from build123d import *

# Parameters (mm, degrees)
SKETCH_R     = 8.5
PAD_DEPTH    = 38
SKETCH001_R  = 4.6
PAD001_DEPTH = 10
FILLET_R     = 1


with BuildPart() as part:
    # Sketch → Pad (new body)
    with BuildSketch(Plane.XY):
        Circle(SKETCH_R)
    extrude(amount=PAD_DEPTH)

    # Sketch001 (on Face2 of Pad) → Pad001 (join)
    with BuildSketch(Plane(origin=(0, 0, 0), x_dir=(1, 0, 0), z_dir=(0, 0, -1))):
        Circle(SKETCH001_R)
    extrude(amount=PAD001_DEPTH)

    # Fillet
    fillet_edges = [part.edges().sort_by_distance(p)[0] for p in [
        (-4.6, 0, -10),
        (-8.5, 0, 0),
    ]]
    fillet(fillet_edges, radius=FILLET_R)


solid = part.part
Build history of the part. All positions in model axes, mm. A direction names the side the tool comes from. Round coordinates to 2 decimals unless told otherwise and drop trailing zeros. Write each loop counter-clockwise with the first axis right and the second up, starting at its lowest first coordinate (ties: lowest second). Pieces come first, ordered by that corner, then holes. Notation, with made-up numbers: M 28.5,79.5 L 66.5,79.5 A26 ccw 66.5,115.5 Z; hole C -36,50 d5. An arc over 180 degrees is marked long. Answer as a JSON object with one key per item and string values. Group by question number.
(1) Cut at C-C (z = 10). Give the cut face in (x, y), and give its area (3 significant figures).
(2) Which spindle directions (+Z, -Z, +X, -X, +Y, -Y) get a long thin tool onto all of the face, cutting with end or side? Do faces 1 (the flat face through (0, 0, -10)), 2 (the flat face through (5, 0, 0)). Say none if no direction does.
(3) Flat gauge pins, fed straight in: pin 1 (1.5 mm diameter, centred on x = 5, z = 31, fed in from +Y); pin 2 (2 mm diameter, centred on x = 5.5, z = 17.5, fed in from +Y); pin 3 (1 mm diameter, centred on x = 5, z = 6, fed in from -Y). Where does each tip first touch, or does it go through?
(4) Drill centre lines: L1, parallel to X at y = -0.25, z = 1; L2, parallel to Z at x = 0, y = -5; L3, parallel to X at y = 4, z = 33.5. Where is each one in solid material? Low to high.
(5) Cut at A-A (x = 0). Give the cut face in (y, z).
Responses:
{
 "1": {"outline": "C 0,0 d17", "area": "227 mm2"},
 "2": {"face 1": "-Z, +X, -X, +Y, -Y", "face 2": "-Z"},
 "3": {"pin 1": "stops at y = 7.36", "pin 2": "stops at y = 7.21", "pin 3": "stops at y = -7.21"},
 "4": {"L1": "x = -8.5 to 8.5", "L2": "z = 0 to 38", "L3": "x = -7.5 to 7.5"},
 "5": {"outline": "M -8.5,1 A1 ccw -7.5,0 L -4.6,0 L -4.6,-9 A1 ccw -3.6,-10 L 3.6,-10 A1 ccw 4.6,-9 L 4.6,0 L 7.5,0 A1 ccw 8.5,1 L 8.5,38 L -8.5,38 Z"}
}
